```python
from build123d import *

# Parameters (mm, degrees)
SKETCH1_R           = 63.5
SKETCH1_R_2         = 50.8
BOSS_EXTRUDE1_DEPTH = 3.175
SKETCH2_R           = 3.175
SKETCH3_R           = 77.7875
SKETCH3_R_2         = 63.5
BOSS_EXTRUDE2_DEPTH = 6.35
SKETCH4_R           = 2.4892
CUT_EXTRUDE1_DEPTH  = 7.35
CIRPATTERN1_COUNT   = 12
BOSS_EXTRUDE3_DEPTH = 6.35
SKETCH6_R           = 31.75
CUT_EXTRUDE2_DEPTH  = 7.35
SKETCH7_R           = 2.5527
CUT_EXTRUDE3_DEPTH  = 7.35
BOSS_EXTRUDE4_DEPTH = 6.35
CUT_EXTRUDE4_DEPTH  = 7.35


with BuildPart() as part:
    # Sketch1 → Boss-Extrude1 (new body, symmetric)
    with BuildSketch(Plane(origin=(0, 0, 0), x_dir=(1, 0, 0), z_dir=(0, 1, 0))):
        Circle(SKETCH1_R)
        Circle(SKETCH1_R_2, mode=Mode.SUBTRACT)
    extrude(amount=BOSS_EXTRUDE1_DEPTH, both=True)

    # Sketch2 → Cut-Revolve1 (revolve, cut)
    with BuildSketch(Plane.XY):
        with Locations((57.15, 3.81)):
            Circle(SKETCH2_R)
    revolve(axis=Axis((0, 0, 0), (0, 1, 0)), mode=Mode.SUBTRACT)

    # Sketch3 → Boss-Extrude2 (add, through all)
    with BuildSketch(Plane.XZ.offset(3.175)):
        Circle(SKETCH3_R)
        Circle(SKETCH3_R_2, mode=Mode.SUBTRACT)
    extrude(amount=-BOSS_EXTRUDE2_DEPTH)

    # Sketch4 → Cut-Extrude1 (cut, through all)
    with BuildSketch(Plane(origin=(0, 3.175, 0), x_dir=(1, 0, 0), z_dir=(0, 1, 0))):
        with Locations((0, -73.025)):
            Circle(SKETCH4_R)
    cut_extrude1 = extrude(amount=-CUT_EXTRUDE1_DEPTH, mode=Mode.SUBTRACT)

    # CirPattern1: Cut-Extrude1 ×12 about axis, 5 skipped
    cirpattern1_axis = Axis((0, 0, 0), (0, 1, 0))
    add([cut_extrude1.rotate(cirpattern1_axis, i * 360 / CIRPATTERN1_COUNT) for i in range(1, CIRPATTERN1_COUNT) if i not in (4, 5, 6, 7, 8)], mode=Mode.SUBTRACT)

    # Sketch5 → Boss-Extrude3 (add, through all)
    with BuildSketch(Plane(origin=(0, 3.175, 0), x_dir=(1, 0, 0), z_dir=(0, 1, 0))):
        with BuildLine():
            Line((74.895357071, 21.013820344), (87.737123324, 33.855586598))
            Line((87.737123324, 33.855586598), (81.001931233, 40.590778688))
            Line((81.001931233, 40.590778688), (71.363979938, 30.952827393))
            ThreePointArc((71.363979938, 30.952827393), (73.298324543, 26.043248173), (74.895357071, 21.013820344))
        make_face()
        with BuildLine():
            Line((-71.363979938, 30.952827393), (-81.001931233, 40.590778688))
            Line((-81.001931233, 40.590778688), (-87.737123324, 33.855586598))
            Line((-87.737123324, 33.855586598), (-74.895357071, 21.013820344))
            ThreePointArc((-74.895357071, 21.013820344), (-73.298324543, 26.043248173), (-71.363979938, 30.952827393))
        make_face()
    extrude(amount=-BOSS_EXTRUDE3_DEPTH)

    # Sketch6 → Cut-Extrude2 (cut, through all)
    with BuildSketch(Plane(origin=(0, 3.175, 0), x_dir=(1, 0, 0), z_dir=(0, 1, 0))):
        with Locations((59.128754095, 77.058092601)):
            Circle(SKETCH6_R)
    cut_extrude2 = extrude(amount=-CUT_EXTRUDE2_DEPTH, mode=Mode.SUBTRACT)

    # Sketch7 → Cut-Extrude3 (cut, through all)
    with BuildSketch(Plane(origin=(0, 3.175, 0), x_dir=(1, 0, 0), z_dir=(0, 1, 0))):
        with Locations((-24.461985581, 65.426552419)):
            Circle(SKETCH7_R)
        with Locations((-60.491874454, 34.925)):
            Circle(SKETCH7_R)
        with Locations((24.461985581, 65.426552419)):
            Circle(SKETCH7_R)
        with Locations((60.491874454, 34.925)):
            Circle(SKETCH7_R)
    extrude(amount=-CUT_EXTRUDE3_DEPTH, mode=Mode.SUBTRACT)

    # Sketch9 → Boss-Extrude4 (add, through all)
    with BuildSketch(Plane(origin=(0, 3.175, 0), x_dir=(1, 0, 0), z_dir=(0, 1, 0))):
        Polygon((75.767612718, 17.611474078), (73.630311762, 19.748775035), (87.737123324, 33.855586598), (89.874424281, 31.718285641), align=None)
        Polygon((81.001931233, 40.590778688), (63.054974858, 45.551787033), (71.363979938, 30.952827393), align=None)
    boss_extrude4 = extrude(amount=-BOSS_EXTRUDE4_DEPTH)

    # Mirror1: Cut-Extrude2, Boss-Extrude4 across plane
    add(cut_extrude2.mirror(Plane(origin=(0, 0, 0), x_dir=(0, 0, 1), z_dir=(1, 0, 0))), mode=Mode.SUBTRACT)
    add(boss_extrude4.mirror(Plane(origin=(0, 0, 0), x_dir=(0, 0, 1), z_dir=(1, 0, 0))))

    # Sketch8 → Cut-Extrude4 (cut, through all)
    with BuildSketch(Plane.XZ.offset(3.175)):
        with BuildLine():
            ThreePointArc((-29.027902052, -66.958527944), (-27.924980023, -68.773522948), (-26.148609279, -69.937632415))
            ThreePointArc((-26.148609279, -69.937632415), (0, -74.666071244), (26.148609279, -69.937632415))
            ThreePointArc((26.148609279, -69.937632415), (27.924980023, -68.773522948), (29.027902052, -66.958527944))
            ThreePointArc((29.027902052, -66.958527944), (28.220438074, -69.795964761), (27.679819148, -72.696098714))
            ThreePointArc((27.679819148, -72.696098714), (0, -77.7875), (-27.679819148, -72.696098714))
            ThreePointArc((-27.679819148, -72.696098714), (-28.220438074, -69.795964761), (-29.027902052, -66.958527944))
        make_face()
    extrude(amount=-CUT_EXTRUDE4_DEPTH, mode=Mode.SUBTRACT)


solid = part.part
```
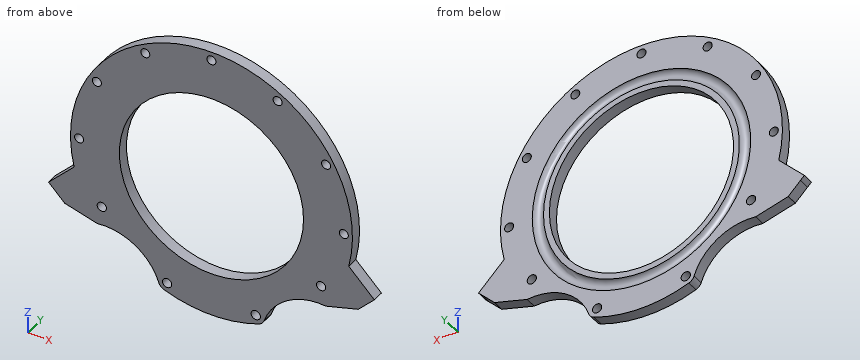
Can you work these out from the model? Positions are in its coordinate system, mm. Give positions to 0.01 mm unless a question says otherwise; leave off trailing zeros. One line per item, written item: value.
1) I want a section at A-A, the plane x = 0. Count the separate pieces of the cut face and the enclosed holes in it, plus the area to 3 significant figures.
Answer sheet:
separate pieces: 3
enclosed holes: 0
area: 268 mm^2
2) For P1, Ø3, axis at x = -45.5, y = -1.5, coming from the -Z side; P2, Ø3, axis at y = 1, z = -29.5, coming from the +X side; P3, Ø1, axis at y = 1, z = 59.5, coming from the -X side, each with a flat end and sliding along its axis, tell me the tip position at first contact or that it passes through.
Answer sheet:
P1: stops at z = -49.14
P2: stops at x = 89.16
P3: stops at x = -50.69
3) Please list where these lines run through material, in increasing order: line 1 along X through (y, z) = (0.5, 0); line 2 along Z through (x, y) = (-18, 1); line 3 along Z through (x, y) = (-61.5, -2.25).
Answer sheet:
line 1: x = -77.79 to -75.51, -70.54 to -50.8, 50.8 to 70.54, 75.51 to 77.79
line 2: z = -72.46 to -55.8, -52.68 to -47.5, 47.5 to 52.68, 55.8 to 75.68
line 3: z = -45.4 to -37.27, -32.58 to 34.73, 38.29 to 47.63
